The model under review builds one solid part; all positions refer to its coordinate system, in mm. Coordinates: 2 decimals unless noted, no trailing zeros. Write each loop counter-clockwise with the first axis right and the second up, starting at its lowest first coordinate (ties: lowest second). Pieces come first, ordered by that corner, then holes. Notation, with made-up numbers: (5.25, 42.25) - (51.25, 42.25) arc R18 cw to (51.25, 53.25) - close; hole circle Ø4 at (-16.75, 22). An arc over 180 degrees is marked (long way). Use one line per item in the form item = value. Start each with the question number.
```python
from build123d import *

# Parameters (mm, degrees)
SKETCH_R   = 17.3
SKETCH_R_2 = 1.5
PAD_DEPTH  = 3


with BuildPart() as part:
    # Sketch → Pad (new body)
    with BuildSketch(Plane.XY):
        with BuildLine():
            ThreePointArc((19.22561, 3.259744), (12.761949, 14.743902), (0.46975, 19.494341))
            ThreePointArc((0.46975, 19.494341), (-3.440809, 23.75207), (-5.982388, 18.559661))
            ThreePointArc((-5.982388, 18.559661), (-14.743902, 12.761949), (-19.22561, 3.259744))
            ThreePointArc((-19.22561, 3.259744), (-24, 0), (-19.22561, -3.259744))
            ThreePointArc((-19.22561, -3.259744), (-12.761949, -14.743902), (-0.46975, -19.494341))
            ThreePointArc((-0.46975, -19.494341), (3.440809, -23.75207), (5.982388, -18.559661))
            ThreePointArc((5.982388, -18.559661), (14.743902, -12.761949), (19.22561, -3.259744))
            ThreePointArc((19.22561, -3.259744), (24, 0), (19.22561, 3.259744))
        make_face()
        Circle(SKETCH_R, mode=Mode.SUBTRACT)
        with Locations((20.5, 0)):
            Circle(SKETCH_R_2, mode=Mode.SUBTRACT)
        with Locations((-20.5, 0)):
            Circle(SKETCH_R_2, mode=Mode.SUBTRACT)
        with Locations((-2.939024, 20.288227)):
            Circle(SKETCH_R_2, mode=Mode.SUBTRACT)
        with Locations((2.939024, -20.288227)):
            Circle(SKETCH_R_2, mode=Mode.SUBTRACT)
    extrude(amount=PAD_DEPTH)


solid = part.part
```
1. Take a section at A-A (x = -20.5). State the section outline as (y, z) points.
2. The part is to be moulded in two halves that separate along X. For faces 1 (the flat face through (-7, -16, 3)), 2 (the cylindrical face through (-24, 0, 1)), say which applies: released by +X, released by -X, zero draft, split by the parting line, or undercut.
3. For P1, Ø1.8, axis at x = 2.94, y = -20.29, coming from the +Z side, flat-tipped, find the tip position at first contact; note if it passes through.
4. Take a section at B-B (y = -9.5). State the section outline as (x, z) points.
5. Take a section at C-C (z = 2.55). State the section outline as (x, y) points, plus the area to 3 significant figures.
6. For L1, parallel to Y at x = -3, z = 1.7; L2, parallel to X at y = -6.5, z = 2.95; L3, parallel to Y at x = 11, z = 2.8, list the stretches that pass through material, from the lowest coordinate up.
Returned:
q1.outline = (-3.5, 0) - (-1.5, 0) - (-1.5, 3) - (-3.5, 3) - close; (1.5, 0) - (3.5, 0) - (3.5, 3) - (1.5, 3) - close
q2.face_1 = zero draft
q2.face_2 = undercut
q3.P1 = through
q4.outline = (-17.03, 0) - (-14.46, 0) - (-14.46, 3) - (-17.03, 3) - close; (14.46, 0) - (17.03, 0) - (17.03, 3) - (14.46, 3) - close
q5.outline = (-19.23, -3.26) arc R19.5 ccw to (-0.47, -19.49) arc R3.5 ccw (long way) to (5.98, -18.56) arc R19.5 ccw to (19.23, -3.26) arc R3.5 ccw (long way) to (19.23, 3.26) arc R19.5 ccw to (0.47, 19.49) arc R3.5 ccw (long way) to (-5.98, 18.56) arc R19.5 ccw to (-19.23, 3.26) arc R3.5 ccw (long way) to start; hole circle Ø3 at (-20.5, 0); hole circle Ø34.6 at (0, 0); hole circle Ø3 at (-2.94, 20.29); hole circle Ø3 at (2.94, -20.29); hole circle Ø3 at (20.5, 0)
q5.area = 333 mm²
q6.L1 = -19.27 to -17.04, 17.04 to 18.79, 21.79 to 23.79
q6.L2 = -18.38 to -16.03, 16.03 to 18.38
q6.L3 = -16.1 to -13.35, 13.35 to 16.1
